Read the model definition and answer for the solid it produces. Units are mm, in the model's axes. A direction names the side the tool comes from. Give positions to 0.01 mm unless a question says otherwise; leave off trailing zeros. Loops run counter-clockwise (first coordinate to the right, second up) from the corner with the lowest first, then second, coordinate; pieces in that order, holes last. Notation, with made-up numbers: (89.25, -39) -> (145.25, -39) arc R21 ccw to (145.25, -28) -> close; hole circle Ø5 at (-6.75, 75.25). An arc over 180 degrees is marked (long way). Return JSON: item names as keys, results as strings. Group by question number.
from build123d import *

# Parameters (mm, degrees)
BOSS_EXTRUDE1_DEPTH = 40
SKETCH2_R           = 6.746805348
CUT_EXTRUDE1_DEPTH  = 40


with BuildPart() as part:
    # Sketch1 → Boss-Extrude1 (new body)
    with BuildSketch(Plane.XY):
        Polygon((-28.677527702, 27.108013937), (-28.677527702, -12.891986063), (-6.677527702, -12.891986063), (-6.677527702, -11.219512195), (-26.677527702, -11.219512195), (-26.677527702, 27.108013937), (-27.701917946, 27.108013937), align=None)
    extrude(amount=BOSS_EXTRUDE1_DEPTH)

    # Sketch2 → Cut-Extrude1 (cut)
    with BuildSketch(Plane.ZY.offset(28.677527702)):
        with Locations((20, 7.108013937)):
            Circle(SKETCH2_R)
    extrude(amount=-CUT_EXTRUDE1_DEPTH, mode=Mode.SUBTRACT)


solid = part.part
1. Straight lines are drawn through the part: line 1 (Y direction, x = -27.85, z = 20); line 2 (Y direction, x = -8.75, z = 17.5); line 3 (X direction, y = 15.5, z = 4). For each, find the intervals that lie inside material, in ascending order. Write a range as from..to.
2. Which of the six approach directions +Z, -Z, +X, -X, +Y, -Y give full straight-line access (tool end or side, diameter ignored) to faces 1 (the flat face through (-26.678, 12, 15)), 2 (the flat face through (-28, 27.108, 20))?
3. Determine the mould class of faces 3 (the flat face through (-27, 3, 0)), 4 (the cylindrical face through (-27.69, 7.4, 13.26)), 5 (the flat face through (-18, -12.892, 20)) for opening direction Y: pulls with the +Y half, pulls with the -Y half, needs draft (parallel to the pull), parting line crosses it, or undercut.
4. Section A-A on z = 20 is taken. Determine the outline of the cut face in (x, y).
5. Flat-ended cylindrical pins translate along their axes: pin 1 Ø1 at (y, z) = (-0.5, 14.5) entering from +X; pin 2 Ø10 at (x, z) = (-19.5, 36) entering from +Y. Find the tip coordinate at first contact, or state that the pin passes through.
6. Section C-C on x = -14.75 is taken. Determine the outline of the cut face in (y, z), then the cut area to 3 significant figures.
7. Section B-B on z = 9 is taken. Determine the outline of the cut face in (x, y).
Completed:
{
 "1": {"line 1": "y = -12.89..0.36, 13.85..27.11", "line 2": "y = -12.89..-11.22", "line 3": "x = -28.68..-26.68"},
 "2": {"face 1": "+Z, -Z, +X, +Y", "face 2": "+Z, -Z, +X, -X, +Y"},
 "3": {"face 3": "needs draft", "face 4": "undercut", "face 5": "pulls with the -Y half"},
 "4": {"outline": "(-28.68, -12.89) -> (-6.68, -12.89) -> (-6.68, -11.22) -> (-26.68, -11.22) -> (-26.68, 0.36) -> (-28.68, 0.36) -> close; (-28.68, 13.85) -> (-26.68, 13.85) -> (-26.68, 27.11) -> (-28.68, 27.11) -> close"},
 "5": {"pin 1": "stops at x = -26.68", "pin 2": "stops at y = -11.22"},
 "6": {"outline": "(-12.89, 0) -> (-11.22, 0) -> (-11.22, 40) -> (-12.89, 40) -> close", "area": "66.9 mm²"},
 "7": {"outline": "(-28.68, -12.89) -> (-6.68, -12.89) -> (-6.68, -11.22) -> (-26.68, -11.22) -> (-26.68, 27.11) -> (-28.68, 27.11) -> close"}
}
